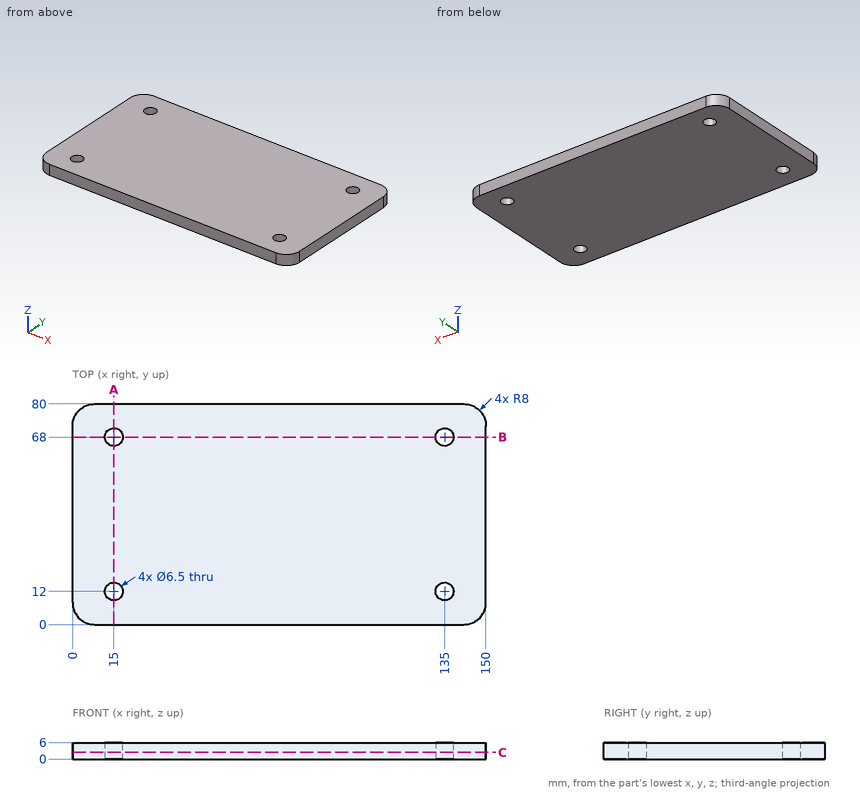
For this review, use the dimensioned drawing (mm, ordinates from the lowest corner) and the shaded views. Coordinates: 2 decimals unless noted, no trailing zeros. Loops run counter-clockwise (first coordinate to the right, second up) from the corner with the lowest first, then second, coordinate; pieces in that order, holes last. Notation, with made-up numbers: (-14.75, 84) -> (-10.75, 84) arc R17 ccw to (-10.75, 92) -> close; hole circle Ø5 at (13, -3). An arc over 180 degrees is marked (long way). Return JSON: item names as keys, results as strings. Group by question number.
(1) For pin 1 Ø10.5 at (x, y) = (15, 68) entering from +Z, flat-tipped, find the tip position at first contact; note if it passes through.
(2) To check wall thickness, follow L1, parallel to Y at x = 135, z = 2.2; L2, parallel to X at y = 68, z = 3.25; L3, parallel to X at y = 4, z = 2. State the ranges of each line that lie inside material, in increasing order.
(3) Consider section C-C, the plane z = 2.4. Give the boundary of the cut face in (x, y).
(4) Consider section A-A, the plane x = 15. Give the boundary of the cut face in (y, z), plus the area to 3 significant figures.
(5) Consider section B-B, the plane y = 68. Give the boundary of the cut face in (x, z).
Results below:
{
 "1": {"pin 1": "stops at z = 6"},
 "2": {"L1": "y = 0 to 8.75, 15.25 to 64.75, 71.25 to 80", "L2": "x = 0 to 11.75, 18.25 to 131.75, 138.25 to 150", "L3": "x = 1.07 to 148.93"},
 "3": {"outline": "(0, 8) arc R8 ccw to (8, 0) -> (142, 0) arc R8 ccw to (150, 8) -> (150, 72) arc R8 ccw to (142, 80) -> (8, 80) arc R8 ccw to (0, 72) -> close; hole circle Ø6.5 at (15, 12); hole circle Ø6.5 at (15, 68); hole circle Ø6.5 at (135, 12); hole circle Ø6.5 at (135, 68)"},
 "4": {"outline": "(0, 0) -> (8.75, 0) -> (8.75, 6) -> (0, 6) -> close; (15.25, 0) -> (64.75, 0) -> (64.75, 6) -> (15.25, 6) -> close; (71.25, 0) -> (80, 0) -> (80, 6) -> (71.25, 6) -> close", "area": "402 mm2"},
 "5": {"outline": "(0, 0) -> (11.75, 0) -> (11.75, 6) -> (0, 6) -> close; (18.25, 0) -> (131.75, 0) -> (131.75, 6) -> (18.25, 6) -> close; (138.25, 0) -> (150, 0) -> (150, 6) -> (138.25, 6) -> close"}
}
